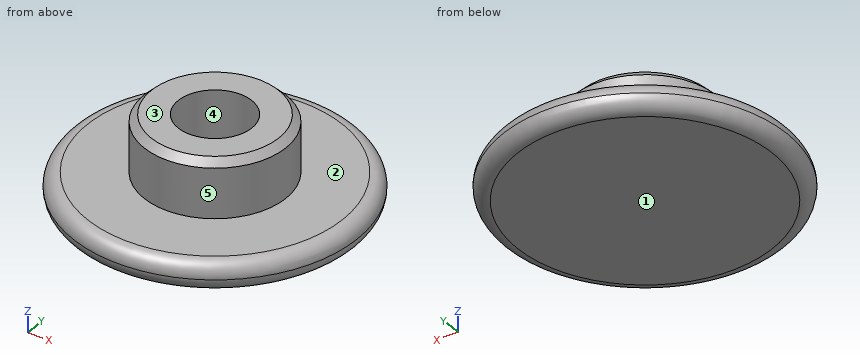
from build123d import *

# Parameters (mm, degrees)
F0_R     = 10
F1_DEPTH = 2
F2_R     = 5
F3_DEPTH = 4
F4_SIZE  = 0.5
F5_R     = 0.99999
F6_R     = 2.6
F7_DEPTH = 3.4


# Not quite as in the source:
# - a fillet or chamfer is up to 0.001 mm smaller than in the source, because OpenCascade refuses the exact size


with BuildPart() as f1:
    # F0 (on Top) → F1 (new body)
    with BuildSketch(Plane.XY):
        Circle(F0_R)
    extrude(amount=F1_DEPTH)

    # F2 (on face) → F3 (join)
    with BuildSketch(Plane.XY.offset(2)):
        Circle(F2_R)
    extrude(amount=F3_DEPTH)

    # F4
    f4_edges = [f1.edges().sort_by_distance(p)[0] for p in [
        (-5, 0, 6),
    ]]
    chamfer(f4_edges, length=F4_SIZE)

    # F5 (radius 1 in the source; OpenCascade refuses exactly that, so slightly less here)
    f5_edges = [f1.edges().sort_by_distance(p)[0] for p in [
        (-10, 0, 0),
        (-10, 0, 2),
    ]]
    fillet(f5_edges, radius=F5_R)

    # F6 (on face) → F7 (cut)
    with BuildSketch(Plane.XY.offset(6)):
        Circle(F6_R)
    extrude(amount=-F7_DEPTH, mode=Mode.SUBTRACT)


solid = f1.part
Model file for the job. Use its own axes, mm. Face numbers are marked on the shaded views. A direction names the side the tool comes from. Give positions to 0.01 mm unless a question says otherwise; leave off trailing zeros. Loops run counter-clockwise (first coordinate to the right, second up) from the corner with the lowest first, then second, coordinate; pieces in that order, holes last.
Item 1: Which spindle directions (+Z, -Z, +X, -X, +Y, -Y) get a long thin tool onto all of the face, cutting with end or side? Do the marked faces 1 and 2. Say none if no direction does.
Check values:
face 1: -Z, +X, -X, +Y, -Y
face 2: +Z
Item 2: Mould opens along Y. For the marked faces 3, 4 and 5 say: +Y half, -Y half, draft (parallel to the pull), parting line (faces both ways), or undercut.
Check values:
face 3: draft
face 4: undercut
face 5: parting line
Item 3: Drop flat-ended pins along their axis: P1, Ø6, axis at x = -6.5, y = 8, coming from the +Z side; P2, Ø1.6, axis at x = 0.5, y = -1, coming from the +Z side; P3, Ø1, axis at y = 1.5, z = 5.5, coming from the -X side. Give the stop position or say it passes through.
Check values:
P1: stops at z = 2
P2: stops at z = 2.6
P3: stops at x = -4.9
Item 4: Drill centre lines: line 1 along Y through (x, z) = (0, 5.05); line 2 along Z through (x, y) = (3.5, -4.25); line 3 along Z through (x, y) = (1.5, 0.75). Where is each one in solid material? Low to high.
Check values:
line 1: y = -5 to -2.6, 2.6 to 5
line 2: z = 0 to 2
line 3: z = 0 to 2.6
Item 5: Slice it at C-C (z = 4.25). Write the cut outline in (x, y).
Check values:
outline: circle Ø10 at (0, 0); hole circle Ø5.2 at (0, 0)
Item 6: Slice it at D-D (z = 2.3). Write the cut outline in (x, y), plus the area to 3 significant figures.
Check values:
outline: circle Ø10 at (0, 0)
area: 78.5 mm2
